Could you check a few things on this model? Use its own coordinates, in mm. Face numbers are marked on the shaded views. A direction names the side the tool comes from. Give positions to 0.01 mm unless a question says otherwise; leave off trailing zeros. Write each loop counter-clockwise with the first axis right and the second up, starting at its lowest first coordinate (ties: lowest second). Pieces come first, ordered by that corner, then holes. Notation, with made-up numbers: M 69,83.5 L 105,83.5 A29 ccw 105,108.5 Z; hole C 8,-13.5 d11. An arc over 180 degrees is marked long. One line per item, written item: value.
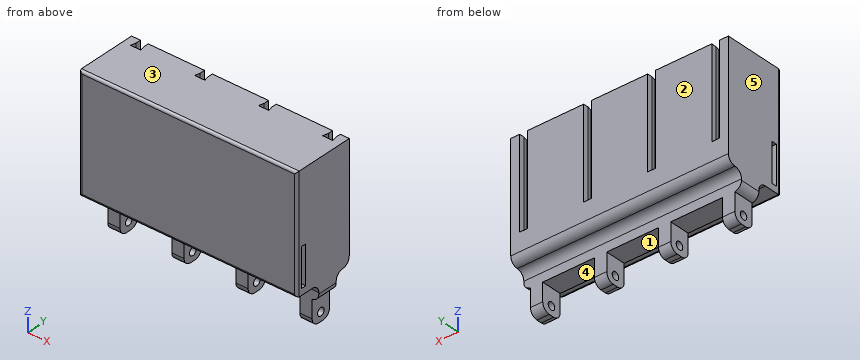
```python
from build123d import *

# Parameters (mm, degrees)
CROQUIS1_R                 = 1.5
SALIENTE_EXTRUIR1_DEPTH    = 42.5
CORTAR_EXTRUIR1_DEPTH      = 78.46128065
CORTAR_EXTRUIR1_DEPTH_BACK = 78.46128065
CROQUIS2_W                 = 2.6
CROQUIS2_H                 = 10
CROQUIS2_W_2               = 20.2
CORTAR_EXTRUIR4_DEPTH      = 78.46128065
CORTAR_EXTRUIR4_DEPTH_BACK = 78.46128065
CROQUIS4_W                 = 15
CROQUIS4_H                 = 2
REDONDEO3_R                = 3
CORTAR_EXTRUIR6_DEPTH      = 35
REDONDEO2_R                = 1


with BuildPart() as part:
    # Croquis1 → Saliente-Extruir1 (new, symmetric)
    with BuildSketch(Plane(origin=(0, 0, 0), x_dir=(0, 0, -1), z_dir=(1, 0, 0))):
        Polygon((-1.5, 9), (-1.5, 1), (-18, 1), (-18, -9), (-63, -9), (-63, 9), (-63, 15), (-18, 15), (-18, 9), align=None)
        with Locations((-5, 5)):
            Circle(CROQUIS1_R, mode=Mode.SUBTRACT)
    extrude(amount=SALIENTE_EXTRUIR1_DEPTH, both=True)

    # Croquis2 → Cortar-Extruir1 (cut, two sides: drawn at the far end of the back side and taken through both)
    with BuildSketch(Plane(origin=(0, 0, 0), x_dir=(1, 0, 0), z_dir=(0, 1, 0)).offset(-CORTAR_EXTRUIR1_DEPTH_BACK)):
        with Locations((-41.2, -6.5)):
            Rectangle(CROQUIS2_W, CROQUIS2_H)
        with Locations((-25, -6.5)):
            Rectangle(CROQUIS2_W_2, CROQUIS2_H)
        with Locations((0, -6.5)):
            Rectangle(CROQUIS2_W_2, CROQUIS2_H)
        with Locations((25, -6.5)):
            Rectangle(CROQUIS2_W_2, CROQUIS2_H)
        with Locations((41.2, -6.5)):
            Rectangle(CROQUIS2_W, CROQUIS2_H)
    extrude(amount=CORTAR_EXTRUIR1_DEPTH + CORTAR_EXTRUIR1_DEPTH_BACK, mode=Mode.SUBTRACT)

    # Croquis4 → Cortar-Extruir4 (cut, two sides: drawn at the far end of the back side and taken through both)
    with BuildSketch(Plane(origin=(0, 0, 0), x_dir=(0, 0, -1), z_dir=(1, 0, 0)).offset(-CORTAR_EXTRUIR4_DEPTH_BACK)):
        with Locations((-28, -6)):
            Rectangle(CROQUIS4_W, CROQUIS4_H)
    extrude(amount=CORTAR_EXTRUIR4_DEPTH + CORTAR_EXTRUIR4_DEPTH_BACK, mode=Mode.SUBTRACT)

    # Redondeo3
    # the kernel refuses this fillet: 3 mm, written as the material it adds along each edge
    with BuildSketch(Plane(origin=(42.5, 1, 18), x_dir=(0, 0, -1), z_dir=(-1, 0, 0)), Plane(origin=(-42.5, 9, 18), x_dir=(0, 0, -1), z_dir=(1, 0, 0))) as redondeo3_piece_1:
        with BuildLine():
            CenterArc((REDONDEO3_R, REDONDEO3_R), REDONDEO3_R, 180, 90)
            Line((0, REDONDEO3_R), (0, 0))
            Line((0, 0), (REDONDEO3_R, 0))
        make_face()
    extrude(amount=85)
    # the kernel refuses this fillet: 3 mm, written as the material it takes off along each edge
    with BuildSketch(Plane(origin=(-47.4, 9, 1.5), x_dir=(0, -1, 0), z_dir=(1, 0, 0)), Plane(origin=(-27.6, 1, 1.5), x_dir=(0, 1, 0), z_dir=(-1, 0, 0))) as redondeo3_2_piece_1:
        with BuildLine():
            CenterArc((REDONDEO3_R, -REDONDEO3_R), REDONDEO3_R, 90, 90)
            Line((0, -REDONDEO3_R), (0, 0))
            Line((0, 0), (REDONDEO3_R, 0))
        make_face()
    extrude(amount=19.8, mode=Mode.SUBTRACT)
    with BuildSketch(Plane(origin=(27.6, 9, 1.5), x_dir=(0, 0, 1), z_dir=(1, 0, 0)), Plane(origin=(47.4, 1, 1.5), x_dir=(0, 0, 1), z_dir=(-1, 0, 0)), Plane(origin=(2.6, 9, 1.5), x_dir=(0, 0, 1), z_dir=(1, 0, 0)), Plane(origin=(22.4, 1, 1.5), x_dir=(0, 0, 1), z_dir=(-1, 0, 0)), Plane(origin=(-22.4, 9, 1.5), x_dir=(0, 0, 1), z_dir=(1, 0, 0)), Plane(origin=(-2.6, 1, 1.5), x_dir=(0, 0, 1), z_dir=(-1, 0, 0))) as redondeo3_2_piece_2:
        with BuildLine():
            CenterArc((REDONDEO3_R, REDONDEO3_R), REDONDEO3_R, 180, 90)
            Line((0, REDONDEO3_R), (0, 0))
            Line((0, 0), (REDONDEO3_R, 0))
        make_face()
    extrude(amount=19.8, mode=Mode.SUBTRACT)
    with BuildSketch(Plane(origin=(42.5, -6.433034374, 11.5), x_dir=(0, 0, 1), z_dir=(0, 1, 0))) as redondeo3_2_piece_3:
        with BuildLine():
            CenterArc((2.973213749, -3), REDONDEO3_R, 90, 82.337744339)
            Line((0, -2.6), (0, 0))
            Line((0, 0), (2.973213749, 0))
        make_face()
    extrude(amount=22.866068747, mode=Mode.SUBTRACT)
    with BuildSketch(Plane(origin=(-42.5, 16.433034374, 11.5), x_dir=(1, 0, 0), z_dir=(0, -1, 0))) as redondeo3_2_piece_4:
        with BuildLine():
            CenterArc((3, 2.973213749), REDONDEO3_R, 180, 82.337744339)
            Line((0, 2.973213749), (0, 0))
            Line((0, 0), (2.6, 0))
        make_face()
    extrude(amount=22.866068747, mode=Mode.SUBTRACT)
    with BuildSketch(Plane(origin=(-50, 15, 18), x_dir=(0, -1, 0), z_dir=(1, 0, 0))) as redondeo3_2_piece_5:
        with BuildLine():
            CenterArc((REDONDEO3_R, -REDONDEO3_R), REDONDEO3_R, 90, 90)
            Line((0, -REDONDEO3_R), (0, 0))
            Line((0, 0), (REDONDEO3_R, 0))
        make_face()
    extrude(amount=100, mode=Mode.SUBTRACT)

    # Croquis5 → Cortar-Extruir6 (cut)
    with BuildSketch(Plane(origin=(0, 0, 63), x_dir=(-1, 0, 0), z_dir=(0, 0, -1))):
        Polygon((11, 13), (10.5, 11), (14.5, 11), (14, 13), (14, 15), (11, 15), align=None)
        Polygon((-39, 13), (-39.5, 11), (-35.5, 11), (-36, 13), (-36, 15), (-39, 15), align=None)
        Polygon((36, 15), (39, 15), (39, 13), (39.5, 11), (35.5, 11), (36, 13), align=None)
        Polygon((-11, 15), (-14, 15), (-14, 13), (-14.5, 11), (-10.5, 11), (-11, 13), align=None)
    extrude(amount=CORTAR_EXTRUIR6_DEPTH, mode=Mode.SUBTRACT)

    # Redondeo2
    redondeo2_edges = [part.edges().sort_by_distance(p)[0] for p in [
        (-42.5, -9, 40.5),
        (0, -9, 18),
        (0, -9, 63),
        (42.5, -9, 40.5),
    ]]
    fillet(redondeo2_edges, radius=REDONDEO2_R)


solid = part.part
```
1) Please list where these lines run through material, in increasing order: L1, parallel to X at y = 3, z = 8.5; L2, parallel to Z at x = -37.3, y = 5; L3, parallel to Y at x = 12, z = 5. Write a range as from..to.
Outcome:
L1: x = -39.9..-35.1, -14.9..-10.1, 10.1..14.9, 35.1..39.9
L2: z = 1.5..3.5, 6.5..63
L3: y = 1..3.5, 6.5..9
2) If we section it at A-A, the plane x = -19.5: Write out the boundary of the cut face in (y, z).
Outcome:
outline: M -9,19 A1 ccw -8,18 L -2,18 A3 cw 1,15 L 1,11.5 L 9,11.5 L 9,15 A3 cw 12,18 A3 ccw 15,21 L 15,63 L -8,63 A1 ccw -9,62 Z; hole M -7,20.5 L -5,20.5 L -5,35.5 L -7,35.5 Z
3) We'd pull the mould along X, two halves only. Please class the marked faces 3, 4 and 5: pulls with the +X half, pulls with the -X half, needs draft (parallel to the pull), parting line crosses it, or undercut.
Outcome:
face 3: needs draft
face 4: undercut
face 5: pulls with the -X half
4) On a 3-axis mill with a long thin cutter (end or side, diameter ignored), from which of +Z, -Z, +X, -X, +Y, -Y can I reach the whole of each face in a straight line? I mean the marked faces 1 and 2. Say none if no direction works.
Outcome:
face 1: -Z, +Y, -Y
face 2: +Z, -Z, +X, -X, +Y
5) I'm going to push flat-ended pins straight in: pin 1 (2.5 mm diameter, centred on y = 4, z = 4.5, fed in from +X); pin 2 (5 mm diameter, centred on y = 5, z = 5, fed in from -X); pin 3 (8 mm diameter, centred on x = -1, y = 11, fed in from -Z); pin 4 (4.5 mm diameter, centred on x = 12.5, y = 13.5, fed in from +Z). Where does each tip first touch, or does it pass through?
Outcome:
pin 1: stops at x = 39.9
pin 2: stops at x = -39.9
pin 3: stops at z = 11.5
pin 4: stops at z = 63
6) If we section it at D-D, the plane y = 5: Give the number of separate pieces and of enclosed holes in the cut face, then the cut area to 3 significant figures.
Outcome:
separate pieces: 5
enclosed holes: 0
area: 4,510 mm^2
7) If we section it at B-B, the plane z = 24.5: Write out the boundary of the cut face in (x, y), then the cut area to 3 significant figures.
Outcome:
outline: M -42.5,-8 A1 ccw -41.5,-9 L 41.5,-9 A1 ccw 42.5,-8 L 42.5,-7 L -42.5,-7 Z; M -42.5,-5 L 42.5,-5 L 42.5,15 L -42.5,15 Z
area: 1,870 mm^2
